Geometry: final body of the model. Coordinates: model frame, mm. Face numbers are marked on the shaded views. A direction names the side the tool comes from. Give positions to 0.01 mm unless a question says otherwise; leave off trailing zeros. Write each loop counter-clockwise with the first axis right and the second up, starting at its lowest first coordinate (ties: lowest second). Pieces come first, ordered by that corner, then holes. Notation, with made-up numbers: (4.5, 13) -> (36.5, 13) arc R15 ccw to (36.5, 21) -> close; hole circle Ø9 at (64, 48.5). An arc over 180 degrees is marked (long way). Use CSV: the item, a comma, the result in double quotes. Start each with the question number.
1) Section B-B (x = 2). Output: boundary loops of the cut face in (y, z), plus the area to 3 significant figures.
2) Set-up query: the marked faces 1 and 2. Return all of +Z, -Z, +X, -X, +Y, -Y with unobstructed straight access to the full face (end or side cutting, diameter ignored); none if empty.
3) Section D-D (x = -3.5). Output: boundary loops of the cut face in (y, z), plus the area to 3 significant figures.
4) Section C-C (z = -5). Output: boundary loops of the cut face in (x, y).
5) Contact query for flat-ended pins moving along their axis: P1, Ø2, axis at x = 0.5, y = 3, coming from the +Z side; P2, Ø0.8, axis at x = 0.5, y = 1, coming from the +Z side; P3, Ø1.3, axis at x = -0.5, z = 7, coming from the +Y side. Output: stop coordinate, or through.
6) Section A-A (y = 1.25). Output: boundary loops of the cut face in (x, z).
7) Material intervals for line 1 (Z direction, x = -1, y = 1.65); line 2 (Z direction, x = 0, y = 0.35); line 3 (Y direction, x = 6.75, z = 1.25), sorted ascending. Write a range as [from, to].
Autodesk Inventor part; units mm, degrees
ref_plane "lens_to_body_XY" through (0, 0, 0) normal (0, 1, 0) x (1, 0, 0)
ref_plane "lens_to_body_YZ" through (0, 0, 0) normal (1, 0, 0) x (0, 0, -1)
ref_plane "lens_to_body_ZX" through (0, 0, 0) normal (0, 0, -1) x (0, 1, 0)
sketch "Sketch_13" plane through (0, 0, 0) normal (0, 0, 1) x (1, 0, 0)
  line L0 (-7.5057, 0) -> (7.5057, 0)
  line L1 (7.5057, 0) -> (7.5057, 5.588)
  line L2 (7.5057, 5.588) -> (-7.5057, 5.588)
  line L3 (-7.5057, 5.588) -> (-7.5057, 0)
extrude "Extrusion1" add sketch "Sketch_13" along normal mid plane 15.0114
sketch "Sketch_21" plane through (0, 0, 0) normal (0, 1, 0) x (-1, 0, 0)
  line L0 (8.89, 8.89) -> (-8.89, 8.89)
  line L1 (-8.89, 8.89) -> (-8.89, -8.89)
  line L2 (-8.89, -8.89) -> (8.89, -8.89)
  line L3 (8.89, -8.89) -> (8.89, 8.89)
  line L4 (7.5057, -7.2517) -> (7.5057, 7.2517)
  arc A0 (7.5057, 7.2517) -> (7.2517, 7.5057) centre (7.2517, 7.2517) ccw
  line L5 (7.2517, 7.5057) -> (-7.2517, 7.5057)
  arc A1 (-7.2517, 7.5057) -> (-7.5057, 7.2517) centre (-7.2517, 7.2517) ccw
  line L6 (-7.5057, 7.2517) -> (-7.5057, -7.2517)
  arc A2 (-7.5057, -7.2517) -> (-7.2517, -7.5057) centre (-7.2517, -7.2517) ccw
  line L7 (-7.2517, -7.5057) -> (7.2517, -7.5057)
  arc A3 (7.2517, -7.5057) -> (7.5057, -7.2517) centre (7.2517, -7.2517) ccw
extrude "Extrusion2" cut sketch "Sketch_21" along normal blind 7.62
sketch "Sketch_14" plane through (0, 0, 0) normal (0, 0, 1) x (1, 0, 0)
  line L0 (-7.5057, 8.128) -> (-7.5057, 4.572)
  line L1 (-7.5057, 4.572) -> (-3.6957, 7.112)
  line L2 (-3.6957, 7.112) -> (3.6957, 7.112)
  line L3 (3.6957, 7.112) -> (7.5057, 4.572)
  line L4 (7.5057, 4.572) -> (7.5057, 8.128)
  line L5 (7.5057, 8.128) -> (-7.5057, 8.128)
extrude "Extrusion3" cut sketch "Sketch_14" along normal mid plane 15.24
sketch "Sketch_15" plane through (0, 0, 0) normal (1, 0, 0) x (0, 1, 0)
  line L0 (8.128, 7.5057) -> (4.572, 7.5057)
  line L1 (4.572, 7.5057) -> (7.112, 3.6957)
  line L2 (7.112, 3.6957) -> (7.112, -3.6957)
  line L3 (7.112, -3.6957) -> (4.572, -7.5057)
  line L4 (4.572, -7.5057) -> (8.128, -7.5057)
  line L5 (8.128, -7.5057) -> (8.128, 7.5057)
extrude "Extrusion4" cut sketch "Sketch_15" along normal mid plane 15.24
sketch "Sketch_17" plane through (0, 0, 7.5057) normal (0, 0, 1) x (1, 0, 0)
  line L0 (-2.54, 0) -> (2.54, 0)
  line L1 (2.54, 0) -> (2.54, 4.064)
  line L2 (2.54, 4.064) -> (-2.54, 4.064)
  line L3 (-2.54, 4.064) -> (-2.54, 0)
extrude "Extrusion5" cut sketch "Sketch_17" against normal blind 0.127
sketch "Sketch_18" plane through (0, 0, 7.5057) normal (0, 0, 1) x (1, 0, 0)
  line L0 (-2.54, 1.524) -> (2.54, 1.524)
  line L1 (2.54, 1.524) -> (2.54, 4.064)
  line L2 (2.54, 4.064) -> (-2.54, 4.064)
  line L3 (-2.54, 4.064) -> (-2.54, 1.524)
extrude "Extrusion6" cut sketch "Sketch_18" against normal blind 0.254
sketch "Sketch_19" plane through (0, 0, 7.5057) normal (0, 0, 1) x (1, 0, 0)
  line L0 (-1.778, 0.508) -> (1.778, 0.508)
  line L1 (1.778, 0.508) -> (1.778, 1.524)
  line L2 (1.778, 1.524) -> (-1.778, 1.524)
  line L3 (-1.778, 1.524) -> (-1.778, 0.508)
extrude "Extrusion7" cut sketch "Sketch_19" against normal blind 1.27
ref_plane "lens_to_body_XY" through (0, 0, 0) normal (0, 1, 0) x (1, 0, 0)
ref_plane "lens_to_body_YZ" through (0, 0, 0) normal (1, 0, 0) x (0, 0, -1)
ref_plane "lens_to_body_ZX" through (0, 0, 0) normal (0, 0, -1) x (0, 1, 0)
properties part number "UB216KKW015C-NR"
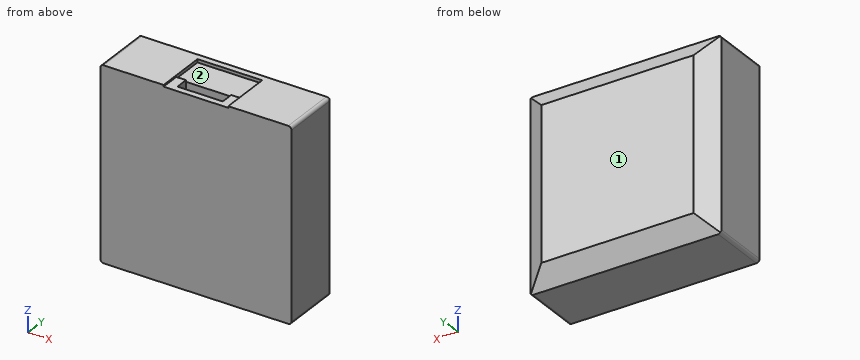
Answers follow:
1,outline,"(0, -7.51) -> (4.57, -7.51) -> (5.59, -5.98) -> (5.59, 5.98) -> (4.57, 7.51) -> (4.06, 7.51) -> (4.06, 7.25) -> (1.52, 7.25) -> (1.52, 7.38) -> (0, 7.38) -> close"
1,area,"81.5 mm^2"
2,face 1,"+Z, -Z, +X, -X, +Y"
2,face 2,"+Z"
3,outline,"(0, -7.51) -> (4.57, -7.51) -> (5.59, -5.98) -> (5.59, 5.98) -> (4.57, 7.51) -> (0, 7.51) -> close"
3,area,"82.3 mm^2"
4,outline,"(-7.51, 0) -> (7.51, 0) -> (7.51, 4.57) -> (5.98, 5.59) -> (-5.98, 5.59) -> (-7.51, 4.57) -> close"
5,P1,"stops at z = 7.25"
5,P2,"stops at z = 6.24"
5,P3,"stops at y = 5.34"
6,outline,"(-7.51, -7.25) arc R0.25 ccw to (-7.25, -7.51) -> (7.25, -7.51) arc R0.25 ccw to (7.51, -7.25) -> (7.51, 7.25) arc R0.25 ccw to (7.25, 7.51) -> (2.54, 7.51) -> (2.54, 7.38) -> (1.78, 7.38) -> (1.78, 6.24) -> (-1.78, 6.24) -> (-1.78, 7.38) -> (-2.54, 7.38) -> (-2.54, 7.51) -> (-7.25, 7.51) arc R0.25 ccw to (-7.51, 7.25) -> close"
7,line 1,"z = [-7.51, 7.25]"
7,line 2,"z = [-7.51, 7.38]"
7,line 3,"y = [0, 5.08]"
